For this review, take the finished solid that the model builds, in its own axes (mm). A direction names the side the tool comes from. Round coordinates to 2 decimals unless told otherwise and drop trailing zeros. Write each loop counter-clockwise with the first axis right and the second up, starting at its lowest first coordinate (ties: lowest second). Pieces come first, ordered by that corner, then holes. Notation, with made-up numbers: (22, -1) -> (46, -1) arc R23 cw to (46, 36) -> close; hole circle Ø6 at (62, 77.5). An arc over 180 degrees is marked (long way). Answer as CSV lines item,"result". Start each with the question number.
Item 1: Take a section at D-D on y = 0. Give the boundary of the cut face in (x, z), then the cut area to 3 significant figures.
Item 2: Wall thickness on probe 1 along X at (y, z) = (-0.25, 0); probe 2 along X at (y, z) = (-0.5, -8); probe 3 along X at (y, z) = (-4.5, -2.5): over which ranges is each line inside the solid? List them lowest first. Write a range as from..to.
Item 3: Mouldability with a two-part tool opening along Z and no side actions: class faces 1 (the cylindrical face through (9.58, -0.17, -11.4)), 2 (the flat face through (10, -7.938, -5)), 3 (the cylindrical face through (0.92, 0.11, 21.19)) as +Z half, -Z half, draft (parallel to the pull), parting line (faces both ways), or undercut.
Item 4: Take a section at A-A on z = 0. Give the boundary of the cut face in (x, y), then the cut area to 3 significant figures.
Item 5: Machinability: for faces 4 (the flat face through (0.762, 2, -17)), 5 (the cylindrical face through (2.48, -0.68, -17.51)), 6 (the cylindrical face through (15.121, 0.055, -5.673)), which of the approach directions +Z, -Z, +X, -X, +Y, -Y give a long, thin tool a straight path to every point of the face, cutting with its end or side? Answer none if there is none.
Item 6: For pin 1 Ø3 at (x, y) = (-3, -1.5) entering from +Z; pin 2 Ø5 at (y, z) = (-6.5, 16.5) entering from +X; pin 3 Ø1 at (y, z) = (1, -1.5) entering from +X; pin 4 Ø8 at (y, z) = (3, 0.5) entering from -X, all flat-tipped, find the tip position at first contact; note any pin that passes through.
Item 7: Take a section at B-B on x = -6.5. Give the boundary of the cut face in (y, z), then the cut area to 3 significant figures.
Item 8: Take a section at C-C on z = -15. Give the boundary of the cut face in (x, y), then the cut area to 3 significant figures.
```python
from build123d import *

# Parameters (mm, degrees)
BOSS_EXTRUDE1_DEPTH        = 7.9375
M3X0_5_TAPPED_HOLE1_REACH  = 50.846
M3X0_5_TAPPED_HOLE1_BORE_R = 1.25
CIRPATTERN1_COUNT          = 3


with BuildPart() as part:
    # Sketch1 → Boss-Extrude1 (new, symmetric)
    with BuildSketch(Plane(origin=(0, 0, 0), x_dir=(1, 0, 0), z_dir=(0, 1, 0))):
        with BuildLine():
            Line((-0.762, 21.195306957), (-0.762, 10.895386179))
            ThreePointArc((-0.762, 10.895386179), (0, -10.922), (0.762, 10.895386179))
            Line((0.762, 10.895386179), (0.762, 21.195306957))
            ThreePointArc((0.762, 21.195306957), (0, -21.209), (-0.762, 21.195306957))
        make_face()
    extrude(amount=BOSS_EXTRUDE1_DEPTH, both=True)

    # Sketch2 → Cut-Revolve1 (revolve, cut)
    with BuildSketch(Plane(origin=(0, 0, 0), x_dir=(1, 0, 0), z_dir=(0, 1, 0)), mode=Mode.PRIVATE) as cut_revolve1_sk:
        Polygon((-16.24122954, 13.6398), (0.762, 13.6398), (0.762, 13.1191), (4.142955705, 13.1191), (4.142955705, 11.39825), (17.885792628, 11.39825), (17.885792628, 15.367), (-16.24122954, 15.367), align=None)
    revolve(cut_revolve1_sk.sketch.rotate(Axis((-16.24122954, 0, -15.367), (-1, 0, 0)), 180), axis=Axis((-16.24122954, 0, -15.367), (-1, 0, 0)), mode=Mode.SUBTRACT)

    # M3x0.5 Tapped Hole1 bore (on position points) → M3x0.5 Tapped Hole1 (cut, up to next)
    with BuildSketch(Plane(origin=(-1.848486148, 0, 21.128293352), x_dir=(0.996194698092, 0, 0.087155742748), z_dir=(-0.087155742748, 0, 0.996194698092)), mode=Mode.PRIVATE) as m3x0_5_tapped_hole1_sk1:
        Circle(M3X0_5_TAPPED_HOLE1_BORE_R)
    m3x0_5_tapped_hole1_tool1 = extrude(m3x0_5_tapped_hole1_sk1.sketch, amount=-M3X0_5_TAPPED_HOLE1_REACH, mode=Mode.PRIVATE) & part.part
    m3x0_5_tapped_hole1 = m3x0_5_tapped_hole1_tool1.solids().sort_by_distance((-1.848486, 0, 21.128293))[0]
    add(m3x0_5_tapped_hole1, mode=Mode.SUBTRACT)

    # CirPattern1: M3x0.5 Tapped Hole1 ×3 about axis
    cirpattern1_axis = Axis((0, 7.9375, 0), (0, -1, 0))
    for i in range(1, CIRPATTERN1_COUNT):
        add(m3x0_5_tapped_hole1.rotate(cirpattern1_axis, i * 360 / CIRPATTERN1_COUNT), mode=Mode.SUBTRACT)


solid = part.part
```
Output values:
1,outline,"(-18.06, -11.12) -> (-9.6, -5.2) arc R10.92 cw to (-2.19, 10.7) -> (-3.09, 20.98) arc R21.21 ccw to start; (-16.63, -13.17) arc R21.21 ccw to (-16.24, -13.64) -> (-0.76, -13.64) -> (-0.76, -10.9) arc R10.92 cw to (-8.17, -7.25) -> close; (-12.55, -17.09) arc R21.21 ccw to (-0.76, -21.2) -> (-0.76, -17.09) -> close; (-0.6, 21.2) -> (0.3, 10.92) arc R10.92 cw to (10.36, -3.45) -> (19.72, -7.81) arc R21.21 ccw to start; (0.76, -21.2) arc R21.21 ccw to (8.71, -19.34) -> (4.14, -19.34) -> (4.14, -17.61) -> (0.76, -17.61) -> close; (0.76, -13.12) -> (4.14, -13.12) -> (4.14, -11.4) -> (17.89, -11.4) arc R21.21 ccw to (18.66, -10.08) -> (9.31, -5.72) arc R10.92 cw to (0.76, -10.9) -> close"
1,area,"803 mm^2"
2,probe 1,"x = -21.21..-10.92, 10.92..21.21"
2,probe 2,"x = -19.64..-13.42, -9.43..-7.44, 7.44..14.45"
2,probe 3,"x = -21.06..-10.63, 10.63..21.06"
3,face 1,"undercut"
3,face 2,"draft"
3,face 3,"parting line"
4,outline,"(-21.21, -7.94) -> (-10.92, -7.94) -> (-10.92, 7.94) -> (-21.21, 7.94) -> close; (10.92, -7.94) -> (21.21, -7.94) -> (21.21, 7.94) -> (10.92, 7.94) -> close"
4,area,"327 mm^2"
5,face 4,"-Z, +Y, -Y"
5,face 5,"+X"
5,face 6,"none"
6,pin 1,"stops at z = 21.16"
6,pin 2,"stops at x = 15.93"
6,pin 3,"stops at x = 21.19"
6,pin 4,"stops at x = -21.21"
7,outline,"(-7.94, -20.19) -> (7.94, -20.19) -> (7.94, -8.78) -> (-7.94, -8.78) -> close; (-7.94, 8.78) -> (7.94, 8.78) -> (7.94, 20.19) -> (-7.94, 20.19) -> close; hole circle Ø3.45 at (0, -15.37)"
7,area,"353 mm^2"
8,outline,"(-14.99, -7.94) -> (-0.76, -7.94) -> (-0.76, -1.69) -> (-14.99, -1.69) -> close; (-14.99, 1.69) -> (-0.76, 1.69) -> (-0.76, 7.94) -> (-14.99, 7.94) -> close; (0.76, -7.94) -> (14.99, -7.94) -> (14.99, -3.95) -> (4.14, -3.95) -> (4.14, -2.22) -> (0.76, -2.22) -> close; (0.76, 2.22) -> (4.14, 2.22) -> (4.14, 3.95) -> (14.99, 3.95) -> (14.99, 7.94) -> (0.76, 7.94) -> close"
8,area,"303 mm^2"
